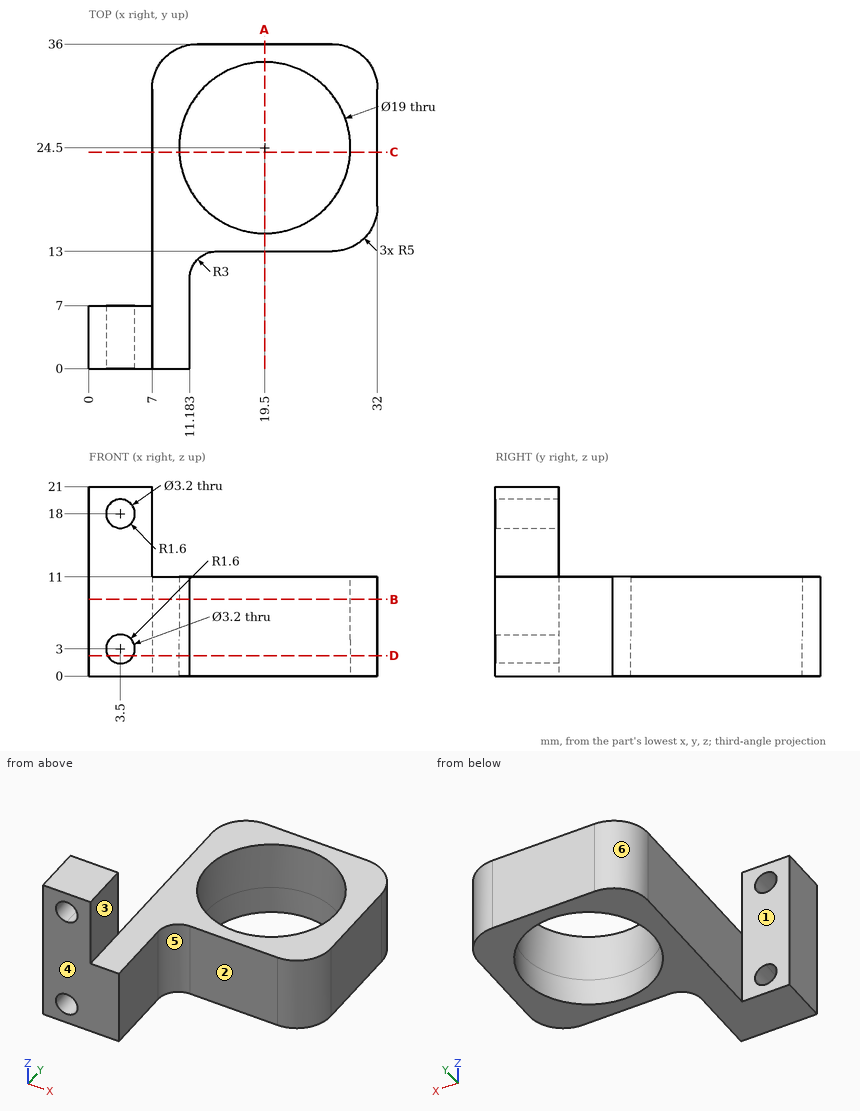
Geometry: see drawing. Coordinates: mm, zero at the bounding-box minimum. A direction names the side the tool comes from. Round coordinates to 2 decimals unless told otherwise and drop trailing zeros. Loops run counter-clockwise (first coordinate to the right, second up) from the corner with the lowest first, then second, coordinate; pieces in that order, holes last. Notation, with made-up numbers: M 67.5,-39 L 72.5,-39 A20 ccw 72.5,-26 Z; hole C 34,-19 d2. An arc over 180 degrees is marked long. Use a Markdown table: item, result. Add a question column.
1. Contact query for flat-ended pins moving along their axis: pin 1 (5.5 mm diameter, centred on y = 18.5, z = 8, fed in from -X); pin 2 (9 mm diameter, centred on x = 23, z = 7, fed in from -Y); pin 3 (2 mm diameter, centred on x = 18, z = 12.5, fed in from +Y); pin 4 (11 mm diameter, centred on y = 5.5, z = 5.5, fed in from +X) (1 decimal). Output: stop coordinate, or through.
2. Ray query, line 1 along Z through (x, y) = (3.5, 5.75); line 2 along Y through (x, z) = (19.5, 2.8); line 3 along X through (y, z) = (9, 3). Return the intervals inside material, ascending. Write a range as [from, to].
3. Cut plane C-C, the plane y = 24. Output: boundary loops of the cut face in (x, z).
4. Set-up query: the marked faces 1, 2 and 3. Return all of +Z, -Z, +X, -X, +Y, -Y with unobstructed straight access to the full face (end or side cutting, diameter ignored); none if empty.
5. Pull-direction query (X, two-part tool) for the marked faces 4, 5 and 6; classes: +X half, -X half, draft (parallel to the pull), parting line (faces both ways), or undercut.
6. Cut plane D-D, the plane z = 2.25. Output: boundary loops of the cut face in (x, y), and give its area (3 significant figures).
7. Cut plane B-B, the plane z = 8.5. Output: boundary loops of the cut face in (x, y).
8. Cut plane A-A, the plane x = 19.5. Output: boundary loops of the cut face in (y, z), and give its area (3 significant figures).
Solution:
| question | item | result |
|---|---|---|
| 1 | pin 1 | stops at x = 7 |
| 1 | pin 2 | stops at y = 13 |
| 1 | pin 3 | passes through |
| 1 | pin 4 | stops at x = 11.4 |
| 2 | line 1 | z = [0, 1.4], [4.6, 16.4], [19.6, 21] |
| 2 | line 2 | y = [13, 15], [34, 36] |
| 2 | line 3 | x = [7, 11.18] |
| 3 | outline | M 7,0 L 10.01,0 L 10.01,11 L 7,11 Z; M 28.99,0 L 32,0 L 32,11 L 28.99,11 Z |
| 4 | face 1 | +Z, -Z, -X, +Y |
| 4 | face 2 | +Z, -Z, +X, -Y |
| 4 | face 3 | +Z, +X, +Y, -Y |
| 5 | face 4 | draft |
| 5 | face 5 | +X half |
| 5 | face 6 | -X half |
| 6 | outline | M 0,0 L 2.09,0 L 2.09,7 L 0,7 Z; M 4.91,0 L 11.18,0 L 11.18,10 A3 cw 14.18,13 L 27,13 A5 ccw 32,18 L 32,31 A5 ccw 27,36 L 12,36 A5 ccw 7,31 L 7,7 L 4.91,7 Z; hole C 19.5,24.5 d19 |
| 6 | area | 361 mm2 |
| 7 | outline | M 0,0 L 11.18,0 L 11.18,10 A3 cw 14.18,13 L 27,13 A5 ccw 32,18 L 32,31 A5 ccw 27,36 L 12,36 A5 ccw 7,31 L 7,7 L 0,7 Z; hole C 19.5,24.5 d19 |
| 8 | outline | M 13,0 L 15,0 L 15,11 L 13,11 Z; M 34,0 L 36,0 L 36,11 L 34,11 Z |
| 8 | area | 44.0 mm2 |
